Check sheet for the modelled part. Datum: model origin and axes. Units: mm. A direction names the side the tool comes from. Give positions to 0.01 mm unless a question says otherwise; leave off trailing zeros. Write each loop counter-clockwise with the first axis right and the second up, starting at its lowest first coordinate (ties: lowest second). Pieces come first, ordered by that corner, then holes. Notation, with made-up numbers: (78, 68.5) -> (135, 68.5) arc R18 cw to (135, 81.5) -> close; hole circle Ø6 at (-13.5, 68.25). An arc over 180 degrees is marked (long way). Answer as a JSON object with one key per item and string values.
from build123d import *

# Parameters (mm, degrees)
SKETCH1_W                = 53
SKETCH1_H                = 15.35
SKETCH1_R                = 1.6
SKETCH1_R_2              = 2.6
BOSS_EXTRUDE1_DEPTH      = 10
BOSS_EXTRUDE2_DEPTH      = 4.325
BOSS_EXTRUDE2_DEPTH_BACK = 19.675
CUT_EXTRUDE1_DEPTH       = 79.033367864
CUT_EXTRUDE2_DEPTH       = 4
SKETCH5_R                = 2.6
BOSS_EXTRUDE3_DEPTH      = 0.4


with BuildPart() as part:
    # Sketch1 → Boss-Extrude1 (new body)
    with BuildSketch(Plane(origin=(0, 0, 0), x_dir=(1, 0, 0), z_dir=(0, 1, 0))):
        with Locations((46.893734614, 0)):
            Rectangle(SKETCH1_W, SKETCH1_H)
        with Locations(Location((52.893734614, 0, 0), (0, 0, 270))):
            Circle(SKETCH1_R, mode=Mode.SUBTRACT)
        with Locations(Location((24.893734614, 0, 0), (0, 0, 270))):
            Circle(SKETCH1_R, mode=Mode.SUBTRACT)
        with Locations(Location((66.393734614, 0, 0), (0, 0, 270))):
            Circle(SKETCH1_R_2, mode=Mode.SUBTRACT)
    extrude(amount=BOSS_EXTRUDE1_DEPTH)

    # Sketch2 → Boss-Extrude2 (add, two sides: drawn at the far end of the back side and taken through both)
    with BuildSketch(Plane(origin=(0, 0, -7.675), x_dir=(-1, 0, 0), z_dir=(0, 0, -1)).offset(-BOSS_EXTRUDE2_DEPTH_BACK)):
        with BuildLine():
            Line((-44.841298991, 14.069078461), (-47.002272565, 16.170952878))
            ThreePointArc((-47.002272565, 16.170952878), (-48.777803829, 13.043328345), (-49.393734614, 9.5))
            Line((-49.393734614, 9.5), (-49.393734614, 0))
            Line((-49.393734614, 0), (-28.393734614, 0))
            Line((-28.393734614, 0), (-28.393734614, 9.5))
            ThreePointArc((-28.393734614, 9.5), (-29.451814157, 14.09348866), (-32.412808532, 17.761210391))
            Line((-32.412808532, 17.761210391), (-34.599781066, 15.649143267))
            ThreePointArc((-34.599781066, 15.649143267), (-37.750161971, 2.087696606), (-44.841298991, 14.069078461))
        make_face()
    extrude(amount=BOSS_EXTRUDE2_DEPTH + BOSS_EXTRUDE2_DEPTH_BACK)

    # Sketch3 → Cut-Extrude1 (cut, through all)
    with BuildSketch(Plane.XY.offset(7.675)):
        with BuildLine():
            Line((46.377049388, 10), (31.410419841, 10))
            ThreePointArc((31.410419841, 10), (38.893734614, 2), (46.377049388, 10))
        make_face()
    extrude(amount=-CUT_EXTRUDE1_DEPTH, mode=Mode.SUBTRACT)

    # Sketch4 → Cut-Extrude2 (cut)
    with BuildSketch(Plane.XZ):
        Polygon((62.410017757, 2.3), (62.410017757, -2.3), (66.393734614, -4.6), (70.377451472, -2.3), (70.377451472, 2.3), (66.393734614, 4.6), align=None)
    extrude(amount=-CUT_EXTRUDE2_DEPTH, mode=Mode.SUBTRACT)

    # Sketch5 → Boss-Extrude3 (add)
    with BuildSketch(Plane.XZ.offset(-4)):
        with Locations(Location((66.393734614, 0, 0), (0, 0, 270))):
            Circle(SKETCH5_R)
    extrude(amount=-BOSS_EXTRUDE3_DEPTH)


solid = part.part
1. Sectioned sample at D-D, the plane y = 14.75. Enter the section's corners in (x, z).
Determined:
{"outline": "(29.8, -12) -> (33.54, -12) -> (33.54, 12) -> (29.8, 12) -> close; (45.54, -12) -> (47.99, -12) -> (47.99, 12) -> (45.54, 12) -> close"}
2. Sectioned sample at A-A, the plane z = 0. Enter the section's corners in (x, y).
Determined:
{"outline": "(20.39, 0) -> (23.29, 0) -> (23.29, 10) -> (20.39, 10) -> close; (26.49, 0) -> (51.29, 0) -> (51.29, 10) -> (49.38, 10) arc R10.5 ccw to (47, 16.17) -> (44.84, 14.07) arc R7.5 cw (long way) to (34.6, 15.65) -> (32.41, 17.76) arc R10.5 ccw to (28.41, 10) -> (26.49, 10) -> close; (54.49, 0) -> (62.41, 0) -> (62.41, 4) -> (70.38, 4) -> (70.38, 0) -> (73.39, 0) -> (73.39, 10) -> (68.99, 10) -> (68.99, 4.4) -> (63.79, 4.4) -> (63.79, 10) -> (54.49, 10) -> close"}
3. Access from +Z, -Z, +X, -X, +Y, -Y to the whole of each face (thin tool, end or side, straight path). Record for faces 1 (the face through (24, 10, -2)), 2 (the face through (28.394, 5, -10)), 3 (the face through (66, 4.4, 0)), 4 (the face through (33.49, 16.72, 0.17)), 5 (the face through (64.43, 1.972, 3.466)).
Determined:
{"face 1": "+Z, -Z, -X, +Y", "face 2": "-Z, -X, +Y, -Y", "face 3": "+Y", "face 4": "+Z, -Z, +Y", "face 5": "-Y"}
4. Sectioned sample at B-B, the plane y = 5.75. Enter the section's corners in (x, z) (3 decimals).
Determined:
{"outline": "(20.394, -7.675) -> (28.394, -7.675) -> (28.394, -12) -> (32.399, -12) -> (32.399, 12) -> (28.394, 12) -> (28.394, 7.675) -> (20.394, 7.675) -> close; (45.389, -12) -> (49.394, -12) -> (49.394, -7.675) -> (73.394, -7.675) -> (73.394, 7.675) -> (49.394, 7.675) -> (49.394, 12) -> (45.389, 12) -> close; hole circle Ø3.2 at (24.894, 0); hole circle Ø3.2 at (52.894, 0); hole circle Ø5.2 at (66.394, 0)"}
5. Mould release check, pull along X, two halves, no side actions. Record for faces 6 (the face through (61, 5, -7.675)), 7 (the face through (49.394, 5, -10)), 8 (the face through (54.243, 4.93, 0.86)), 9 (the face through (45.9, 15.1, 0.2)): released by +X, released by -X, zero draft, split by the parting line, or undercut.
Determined:
{"face 6": "zero draft", "face 7": "released by +X", "face 8": "undercut", "face 9": "undercut"}
6. Sectioned sample at C-C, the plane z = 9. Enter the section's corners in (x, y).
Determined:
{"outline": "(28.39, 0) -> (49.39, 0) -> (49.39, 9.5) arc R10.5 ccw to (47, 16.17) -> (44.84, 14.07) arc R7.5 cw (long way) to (34.6, 15.65) -> (32.41, 17.76) arc R10.5 ccw to (28.39, 9.5) -> close"}
7. Go/stop test with flat-tipped pins: P1, Ø12.5, axis at x = 61, z = -0.5, coming from the +Y side; P2, Ø1.5, axis at y = 16, z = -4.5, coming from the +X side; P3, Ø7, axis at x = 66.39, z = 0, coming from the -Y side. Record where each tip stops, or that it passes through.
Determined:
{"P1": "y = 10", "P2": "x = 47.68", "P3": "y = 4"}
8. Scan lines: L1, parallel to X at y = 9.5, z = -4.25; L2, parallel to X at y = 3.5, z = -4.5; L3, parallel to X at y = 3.5, z = 1.75. Record each from-to range of solid material in increasing order. Write a range as [from, to].
Determined:
{"L1": "[20.39, 31.39], [46.39, 73.39]", "L2": "[20.39, 34.39], [43.39, 66.22], [66.57, 73.39]", "L3": "[20.39, 34.39], [43.39, 62.41], [70.38, 73.39]"}
